Source: CAD feature listing. Evaluate the final solid. Frame: model axes, mm. Round coordinates to 2 decimals unless told otherwise and drop trailing zeros. Write each loop counter-clockwise with the first axis right and the second up, starting at its lowest first coordinate (ties: lowest second). Pieces come first, ordered by that corner, then holes. Notation, with made-up numbers: (1, 42) -> (53, 42) arc R37 ccw to (53, 81) -> close; hole circle Ø7 at (21, 40). An arc over 180 degrees is marked (long way). Put each result on its own line as item: value.
Autodesk Inventor part; units mm, degrees
ref_plane "Work Plane1" through (26, 0, 0) normal (1, 0, 0) x (0, 1, 0)
ref_plane "YZ Plane" through (0, 0, 0) normal (1, 0, 0) x (0, 1, 0)
ref_plane "XZ Plane" through (0, 0, 0) normal (0, 1, 0) x (-1, 0, 0)
sketch "Sketch1" plane through (0, 0, 0) normal (0, 0, 1) x (1, 0, 0)
  line L0 (0, 0) -> (0, 5)
  line L1 (0, 5) -> (26, 5)
  line L2 (26, 5) -> (26, 4.497)
  line L3 (26, 4.497) -> (39, 4.497)
  line L4 (39, 4.497) -> (39, 5)
  line L5 (39, 5) -> (65, 5)
  line L6 (65, 5) -> (65, 0)
  line L7 (65, 0) -> (0, 0)
  dimension "d1" = 10
  dimension "d3" = 8.994
  dimension "d4" = 26
  dimension "d6" = 26
  dimension "d43" = 65
revolve "Вращение1" add sketch "Sketch1" angle 360 about axis through (65, 0, 0) along (-1, 0, 0)
thread "Резьба1"
thread "Резьба2"
chamfer "Фаска1" distance 0.6 angle 45 2 edges at (0, -5, 0) (65, -5, 0)
chamfer "Фаска2" distance 0.4 angle 45 2 edges at (26, -5, 0) (39, -5, 0)
ref_plane "Work Plane1" through (26, 0, 0) normal (1, 0, 0) x (0, 1, 0)
sketch "Sketch2" plane through (26, 0, 0) normal (1, 0, 0) x (0, 1, 0)
  circle A0 centre (0, 0) radius 5
  point P0 (0, 0)
  dimension "d35" = 10
boundary_patch "Участок поверхности1"
equation "\"d8\" = b"
equation "\"d29\" = b"
equation "\"d31\" = C_"
equation "\"d37\" = C2_"
equation "\"d1\" = d"
equation "\"d3\" = d2"
equation "\"d4\" = b"
equation "\"d6\" = b"
equation "\"d43\" = L"
equation "\"d35\" = d"
equation "\"C_\" = 0.6"
equation "\"d\" = 10"
equation "\"d2\" = 8.994"
equation "\"L\" = 65"
equation "\"b\" = 26"
equation "\"d34\" = -b"
equation "\"C2_\" = 0.4"
equation "\"Grip_Length\" = 13"
properties part number "Шпилька 2 M10-6g×65 ГОСТ 22042-76" material "Сталь, мягкая"
Q1. Draft query along X for faces 1 (the flat face through (65, 0, 0)), 2 (the flat face through (0, 0, 0)), 3 (the cylindrical face through (32.591, 4.154, -1.722)), 4 (the cylindrical face through (13.28, -1.08, -4.88)). Return one class per face: +X half, -X half, draft (parallel to the pull), parting line (faces both ways), or undercut.
Ans:
face 1: +X half
face 2: -X half
face 3: undercut
face 4: draft
Q2. Material intervals for line 1 (Z direction, x = 47.5, y = 0.25); line 2 (Z direction, x = 37, y = -0.25), sorted ascending. Write a range as [from, to].
Ans:
line 1: z = [-4.99, 4.99]
line 2: z = [-4.49, 4.49]
Q3. Cut plane A-A on y = 0. Output: boundary loops of the cut face in (x, z).
Ans:
outline: (0, -4.4) -> (0.6, -5) -> (25.6, -5) -> (26, -4.6) -> (26, -4.5) -> (39, -4.5) -> (39, -4.6) -> (39.4, -5) -> (64.4, -5) -> (65, -4.4) -> (65, 4.4) -> (64.4, 5) -> (39.4, 5) -> (39, 4.6) -> (39, 4.5) -> (26, 4.5) -> (26, 4.6) -> (25.6, 5) -> (0.6, 5) -> (0, 4.4) -> close
Q4. Cut plane C-C on x = 13.5. Output: boundary loops of the cut face in (y, z), and give its area (3 significant figures).
Ans:
outline: circle Ø10 at (0, 0)
area: 78.5 mm^2
Q5. Pin query (flat end, axial travel): pin 1 (1.5 mm diameter, centred on x = 47, y = -1, fed in from -Z). Return the tip coordinate at first contact, or that it passes through.
Ans:
pin 1: stops at z = -4.99
